Could you check a few things on this model? Use its own coordinates, in mm. A direction names the side the tool comes from. Coordinates: 2 decimals unless noted, no trailing zeros. Write each loop counter-clockwise with the first axis right and the second up, starting at its lowest first coordinate (ties: lowest second). Pieces come first, ordered by that corner, then holes.
```python
from build123d import *

# Parameters (mm, degrees)
SKETCH1_W           = 12
SKETCH1_H           = 45
SKETCH1_R           = 2.5
BOSS_EXTRUDE1_DEPTH = 2
FILLET3_R           = 5
SKETCH2_W           = 12
SKETCH2_H           = 2
BOSS_EXTRUDE2_DEPTH = 33
SKETCH3_R           = 2.5
CUT_EXTRUDE1_DEPTH  = 33
FILLET4_R           = 5


with BuildPart() as part:
    # Sketch1 → Boss-Extrude1 (new body)
    with BuildSketch(Plane.XY):
        Rectangle(SKETCH1_W, SKETCH1_H)
        with Locations((0, -7.5)):
            Circle(SKETCH1_R, mode=Mode.SUBTRACT)
        with Locations((0, 17.5)):
            Circle(SKETCH1_R, mode=Mode.SUBTRACT)
    extrude(amount=BOSS_EXTRUDE1_DEPTH)

    # Fillet3
    fillet3_edges = [part.edges().sort_by_distance(p)[0] for p in [
        (-6, 22.5, 1),
        (6, 22.5, 1),
    ]]
    fillet(fillet3_edges, radius=FILLET3_R)

    # Sketch2 → Boss-Extrude2 (add)
    with BuildSketch(Plane.XY.offset(2)):
        with Locations((0, -21.5)):
            Rectangle(SKETCH2_W, SKETCH2_H)
    extrude(amount=BOSS_EXTRUDE2_DEPTH)

    # Sketch3 → Cut-Extrude1 (cut)
    with BuildSketch(Plane(origin=(0, -20.5, 0), x_dir=(1, 0, 0), z_dir=(0, 1, 0))):
        with Locations((0, -13)):
            Circle(SKETCH3_R)
        with Locations((0, -29)):
            Circle(SKETCH3_R)
    extrude(amount=-CUT_EXTRUDE1_DEPTH, mode=Mode.SUBTRACT)

    # Fillet4
    fillet4_edges = [part.edges().sort_by_distance(p)[0] for p in [
        (-6, -21.5, 35),
        (6, -21.5, 35),
    ]]
    fillet(fillet4_edges, radius=FILLET4_R)


solid = part.part
```
Item 1: If we mould it in two halves opening along X, with no side actions, what happens to faces 3 (the cylindrical face through (-0.54, -21.49, 15.44)), 4 (the flat face through (6, -8.5, 1.6)), 5 (the cylindrical face through (-0.54, -9.94, 0.99)), 6 (the flat face through (0, -22.5, 17))? For each: released by +X, released by -X, zero draft, split by the parting line, or undercut.
Item 2: Will these pins go through, and if not, where does the flat tip stop? pin 1 Ø2 at (x, y) = (-2.5, -6) entering from +Z; pin 2 Ø5 at (x, z) = (1, 16.5) entering from +Y.
Item 3: I want a section at C-C, the plane y = -6.5. List the corners of the cut face in (x, z) for me.
Item 4: If I drill on line 1 along Y through (x, z) = (0, 1.1); line 2 along Z through (x, y) = (0, -20.9); line 3 along X through (y, z) = (-21.55, 13), over which ranges is the centre line in solid material (lowest first)?
Item 5: I want a section at B-B, the plane x = 0. List the corners of the cut face in (y, z) for me, then the cut area to 3 significant figures.
Item 6: I want a section at A-A, the plane z = 13. List the corners of the cut face in (x, y) for me, then the cut area to 3 significant figures.
Item 7: I want a section at D-D, the plane y = 0.5. List the corners of the cut face in (x, z) for me, then the cut area to 3 significant figures.
Item 8: Which directions (+Z, -Z, +X, -X, +Y, -Y) give clear straight access to the entire face, cutting with the end or side of a thin tool? Please do faces 1 (the flat face through (0, 1, 2)), 2 (the flat face through (0, 22.5, 1)).
Taken from the geometry:
1. face 3: undercut
1. face 4: released by +X
1. face 5: undercut
1. face 6: zero draft
2. pin 1: stops at z = 2
2. pin 2: stops at y = -20.5
3. outline: (-6, 0) - (-2.29, 0) - (-2.29, 2) - (-6, 2) - close; (2.29, 0) - (6, 0) - (6, 2) - (2.29, 2) - close
4. line 1: y = -22.5 to -10, -5 to 15, 20 to 22.5
4. line 2: z = 0 to 10.5, 15.5 to 26.5, 31.5 to 35
4. line 3: x = -6 to -2.5, 2.5 to 6
5. outline: (-22.5, 0) - (-10, 0) - (-10, 2) - (-20.5, 2) - (-20.5, 10.5) - (-22.5, 10.5) - close; (-22.5, 15.5) - (-20.5, 15.5) - (-20.5, 26.5) - (-22.5, 26.5) - close; (-22.5, 31.5) - (-20.5, 31.5) - (-20.5, 35) - (-22.5, 35) - close; (-5, 0) - (15, 0) - (15, 2) - (-5, 2) - close; (20, 0) - (22.5, 0) - (22.5, 2) - (20, 2) - close
5. area: 116 mm2
6. outline: (-6, -22.5) - (-2.5, -22.5) - (-2.5, -20.5) - (-6, -20.5) - close; (2.5, -22.5) - (6, -22.5) - (6, -20.5) - (2.5, -20.5) - close
6. area: 14.0 mm2
7. outline: (-6, 0) - (6, 0) - (6, 2) - (-6, 2) - close
7. area: 24.0 mm2
8. face 1: +Z, +X, -X, +Y
8. face 2: +Z, -Z, +X, -X, +Y
